```python
from build123d import *

# Parameters (mm, degrees)
BOSS_EXTRUDE1_DEPTH = 1.651
CUT_EXTRUDE1_DEPTH  = 4.302


with BuildPart() as part:
    # Sketch1 → Boss-Extrude1 (new body, symmetric)
    with BuildSketch(Plane.XY):
        Polygon((85.181948, -17.8435), (85.181948, 17.8435), (65.084948, 17.8435), (65.084948, -2.54), (61.782948, -2.54), (61.782948, 17.8435), (-61.782948, 17.8435), (-61.782948, -2.54), (-65.084948, -2.54), (-65.084948, 17.8435), (-85.181948, 17.8435), (-85.181948, -17.8435), align=None)
    extrude(amount=BOSS_EXTRUDE1_DEPTH, both=True)

    # Sketch2 → Cut-Extrude1 (cut, through all)
    with BuildSketch(Plane.XY.offset(1.651)):
        Polygon((85.181948, 2.667), (80.101948, 2.667), (80.101948, 4.445), (74.513948, 4.445), (74.513948, 2.667), (67.401948, 2.667), (67.401948, -2.667), (74.513948, -2.667), (74.513948, -4.445), (80.101948, -4.445), (80.101948, -2.667), (85.181948, -2.667), align=None)
        Polygon((-85.181948, -2.667), (-80.101948, -2.667), (-80.101948, -4.445), (-74.513948, -4.445), (-74.513948, -2.667), (-67.401948, -2.667), (-67.401948, 2.667), (-74.513948, 2.667), (-74.513948, 4.445), (-80.101948, 4.445), (-80.101948, 2.667), (-85.181948, 2.667), align=None)
    extrude(amount=-CUT_EXTRUDE1_DEPTH, mode=Mode.SUBTRACT)


solid = part.part
```
Geometry check sheet. Reference: the model listing, model coordinates, mm. A direction names the side the tool comes from. Round coordinates to 2 decimals unless told otherwise and drop trailing zeros. Write each loop counter-clockwise with the first axis right and the second up, starting at its lowest first coordinate (ties: lowest second). Pieces come first, ordered by that corner, then holes. Notation, with made-up numbers: (38.5, -35) -> (58.5, -35) arc R12 cw to (58.5, -16) -> close; hole circle Ø9 at (-19.5, 0). An arc over 180 degrees is marked (long way). Put each result on its own line as item: value.
1) Access from +Z, -Z, +X, -X, +Y, -Y to the whole of each face (thin tool, end or side, straight path). Record for faces 5 (the face through (71, 2.667, 0)), 6 (the face through (85.182, 10, 0)), 7 (the face through (-77, -4.445, 0)), 8 (the face through (63, -2.54, 0)), 9 (the face through (-83, -2.667, 0)).
Recorded:
face 5: +Z, -Z, +X
face 6: +Z, -Z, +X, +Y, -Y
face 7: +Z, -Z
face 8: +Z, -Z, +Y
face 9: +Z, -Z, -X
2) Thickness scan on probe 1 along X at (y, z) = (11, -0.75); probe 2 along X at (y, z) = (-3.5, 0.7); probe 3 along Y at (x, z) = (77, -1.5) (1 decimal). Record the ranges inside material, lowest first. Write a range as from..to.
Recorded:
probe 1: x = -85.18..-65.08, -61.78..61.78, 65.08..85.18
probe 2: x = -85.18..-80.1, -74.51..74.51, 80.1..85.18
probe 3: y = -17.8..-4.4, 4.4..17.8
3) Release check for a two-part mould opening along Y. For faces 1 (the face through (-65.085, 8, 0)), 2 (the face through (-1, -17.844, 0)), 3 (the face through (75, 17.844, 0)), 4 (the face through (77, 4.445, 0)) record: pulls with the +Y half, pulls with the -Y half, needs draft (parallel to the pull), parting line crosses it, or undercut.
Recorded:
face 1: needs draft
face 2: pulls with the -Y half
face 3: pulls with the +Y half
face 4: undercut
4) Cross-section at A-A, the plane y = 15. Enter the section's corners in (x, z).
Recorded:
outline: (-85.18, -1.65) -> (-65.08, -1.65) -> (-65.08, 1.65) -> (-85.18, 1.65) -> close; (-61.78, -1.65) -> (61.78, -1.65) -> (61.78, 1.65) -> (-61.78, 1.65) -> close; (65.08, -1.65) -> (85.18, -1.65) -> (85.18, 1.65) -> (65.08, 1.65) -> close
5) Depth check by flat-ended pin: P1, Ø1.7, axis at x = 64, z = 0.5, coming from the +Y side; P2, Ø1.7, axis at y = -0.5, z = -0.5, coming from the -X side. Enter the tip coordinate at first touch or a pass-through.
Recorded:
P1: stops at y = -2.54
P2: stops at x = -67.4
6) Cross-section at B-B, the plane x = 70. Enter the section's corners in (y, z).
Recorded:
outline: (-17.84, -1.65) -> (-2.67, -1.65) -> (-2.67, 1.65) -> (-17.84, 1.65) -> close; (2.67, -1.65) -> (17.84, -1.65) -> (17.84, 1.65) -> (2.67, 1.65) -> close
